Source: CAD feature listing. Evaluate the final solid. Frame: model axes, mm. Face numbers are marked on the shaded views. Round coordinates to 2 decimals unless told otherwise and drop trailing zeros. Write each loop counter-clockwise with the first axis right and the second up, starting at its lowest first coordinate (ties: lowest second). Pieces come first, ordered by that corner, then holes. Notation, with made-up numbers: M 62.25,75.5 L 120.25,75.5 A9 ccw 120.25,91.5 Z; hole C 14,5.25 d3. An arc over 180 degrees is marked long. Use a Markdown table: item, result.
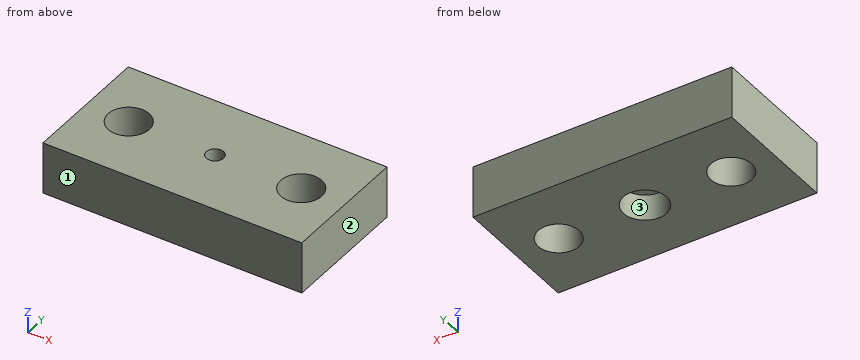
```python
from build123d import *

# Parameters (mm, degrees)
SKETCH1_W           = 30
SKETCH1_H           = 15
SKETCH1_R           = 1
SKETCH1_R_2         = 2.38125
BOSS_EXTRUDE1_DEPTH = 6
SKETCH3_R           = 2.5
CUT_EXTRUDE2_DEPTH  = 3


with BuildPart() as part:
    # Sketch1 → Boss-Extrude1 (new body)
    with BuildSketch(Plane.XY):
        Rectangle(SKETCH1_W, SKETCH1_H)
        Circle(SKETCH1_R, mode=Mode.SUBTRACT)
        with Locations((10, 0)):
            Circle(SKETCH1_R_2, mode=Mode.SUBTRACT)
        with Locations((-10, 0)):
            Circle(SKETCH1_R_2, mode=Mode.SUBTRACT)
    extrude(amount=BOSS_EXTRUDE1_DEPTH)

    # Sketch3 → Cut-Extrude2 (cut)
    with BuildSketch(Plane(origin=(0, 0, 0), x_dir=(-1, 0, 0), z_dir=(0, 0, -1))):
        Circle(SKETCH3_R)
    extrude(amount=-CUT_EXTRUDE2_DEPTH, mode=Mode.SUBTRACT)


solid = part.part
```
Q1. Section B-B on y = 0. Return loops of the section in (x, z).
Results are:
| item | result |
|---|---|
| outline | M -15,0 L -12.38,0 L -12.38,6 L -15,6 Z; M -7.62,0 L -2.5,0 L -2.5,3 L -1,3 L -1,6 L -7.62,6 Z; M 1,3 L 2.5,3 L 2.5,0 L 7.62,0 L 7.62,6 L 1,6 Z; M 12.38,0 L 15,0 L 15,6 L 12.38,6 Z |
Q2. Line query: L1, parallel to Y at x = 0, z = 2.1; L2, parallel to X at y = 2, z = 4.15; L3, parallel to Y at x = -10, z = 3.05. Output: solid intervals per line, ascending.
Results are:
| item | result |
|---|---|
| L1 | -7.5 to -2.5, 2.5 to 7.5 |
| L2 | -15 to -11.29, -8.71 to 8.71, 11.29 to 15 |
| L3 | -7.5 to -2.38, 2.38 to 7.5 |
Q3. Section D-D on x = -1.5. Return loops of the section in (y, z), plus the area to 3 significant figures.
Results are:
| item | result |
|---|---|
| outline | M -7.5,0 L -2,0 L -2,3 L 2,3 L 2,0 L 7.5,0 L 7.5,6 L -7.5,6 Z |
| area | 78.0 mm^2 |
Q4. Mould query, pull axis X, two halves, no side actions, for the marked faces 1, 2 and 3. Classes: +X half, -X half, draft (parallel to the pull), parting line (faces both ways), or undercut.
Results are:
| item | result |
|---|---|
| face 1 | draft |
| face 2 | +X half |
| face 3 | undercut |
Q5. First-contact query: pin 1 Ø4 at (x, y) = (10, 0) entering from +Z; pin 2 Ø1.5 at (x, y) = (0, 0.5) entering from -Z. Flat tips, straight axial feed; report the tip coordinate or a pass-through.
Results are:
| item | result |
|---|---|
| pin 1 | through |
| pin 2 | z = 3 |
Q6. Section C-C on z = 2.25. Return loops of the section in (x, y).
Results are:
| item | result |
|---|---|
| outline | M -15,-7.5 L 15,-7.5 L 15,7.5 L -15,7.5 Z; hole C -10,0 d4.76; hole C 0,0 d5; hole C 10,0 d4.76 |
Q7. Section A-A on x = -10. Return loops of the section in (y, z).
Results are:
| item | result |
|---|---|
| outline | M -7.5,0 L -2.38,0 L -2.38,6 L -7.5,6 Z; M 2.38,0 L 7.5,0 L 7.5,6 L 2.38,6 Z |
